Here's how the part is built. I have some questions about the finished solid (model axes, mm). Give positions to 0.01 mm unless a question says otherwise; leave off trailing zeros. Use a Markdown table: item, result.
```python
from build123d import *

# Parameters (mm, degrees)
SKETCH1_R           = 17.4625
SKETCH1_R_2         = 14.4145
BOSS_EXTRUDE1_DEPTH = 1070
SKETCH2_R           = 1.5
CUT_EXTRUDE2_DEPTH  = 1070
CIRPATTERN1_COUNT   = 16


with BuildPart() as part:
    # Sketch1 → Boss-Extrude1 (new body)
    with BuildSketch(Plane(origin=(0, 0, 0), x_dir=(1, 0, 0), z_dir=(0, 1, 0))):
        with Locations(Location((0, 0, 0), (0, 0, 270))):
            Circle(SKETCH1_R)
        with Locations(Location((0, 0, 0), (0, 0, 270))):
            Circle(SKETCH1_R_2, mode=Mode.SUBTRACT)
    extrude(amount=BOSS_EXTRUDE1_DEPTH)

    # Sketch2 → Cut-Extrude2 (cut, symmetric)
    with BuildSketch(Plane(origin=(0, 0, 0), x_dir=(1, 0, 0), z_dir=(0, 1, 0))):
        with Locations((17.4625, 0)):
            Circle(SKETCH2_R)
    cut_extrude2 = extrude(amount=CUT_EXTRUDE2_DEPTH, both=True, mode=Mode.SUBTRACT)

    # CirPattern1: Cut-Extrude2 ×16 about axis
    cirpattern1_axis = Axis((0, 0, 0), (0, 1, 0))
    for i in range(1, CIRPATTERN1_COUNT):
        add(cut_extrude2.rotate(cirpattern1_axis, i * 360 / CIRPATTERN1_COUNT), mode=Mode.SUBTRACT)


solid = part.part
```
Item 1: Will these pins go through, and if not, where does the flat tip stop? pin 1 Ø4 at (y, z) = (880.5, -6) entering from +X; pin 2 Ø6 at (x, y) = (11.5, 650.5) entering from -Z; pin 3 Ø2 at (y, z) = (929.5, -8.5) entering from -X.
Values:
| item | result |
|---|---|
| pin 1 | stops at x = 17 |
| pin 2 | stops at z = -15.25 |
| pin 3 | stops at x = -15.5 |
Item 2: Thinking about a two-plate mould opening in X: for faces 1 (the cylindrical face through (-14.072, 527.51, -3.125)), 2 (the flat face through (7, 1070, -13)), which applies, +X half, -X half, draft (parallel to the pull), parting line (faces both ways), or undercut?
Values:
| item | result |
|---|---|
| face 1 | undercut |
| face 2 | draft |
Item 3: I need wall thicknesses on line 1 along X through (y, z) = (805, 0); line 2 along Z through (x, y) = (11, 744); line 3 along Z through (x, y) = (15, 399). Which ranges of each line are inside material? Lowest first, please. Write a range as [from, to].
Values:
| item | result |
|---|---|
| line 1 | x = [-15.96, -14.41], [14.41, 15.96] |
| line 2 | z = [-13.56, -13.01], [-11.69, -9.32], [9.32, 11.69], [13.01, 13.56] |
| line 3 | z = [-8.94, -7.67], [-5.7, 5.7], [7.67, 8.94] |
